```python
from build123d import *

# Parameters (mm, degrees)
BOSS_EXTRU_1_DEPTH           = 23
BOSS_EXTRU_2_DEPTH           = 55.74
ENL_V_MAT_EXTRU_2_DEPTH      = 166.850257131
ENL_V_MAT_EXTRU_2_DEPTH_BACK = 166.850257131
ENL_V_MAT_EXTRU_3_DEPTH      = 172.327320122
ENL_V_MAT_EXTRU_3_DEPTH_BACK = 172.327320122


with BuildPart() as part:
    # Esquisse1 → Boss.-Extru.1 (new body)
    with BuildSketch(Plane.XY):
        with BuildLine():
            Line((39.457988868, 163.966514235), (39.457988868, 111.179894524))
            ThreePointArc((39.457988868, 111.179894524), (40.679417093, 109.678629524), (41.957988868, 108.225722877))
            Line((41.957988868, 108.225722877), (41.957988868, 163.966514235))
            Line((41.957988868, 163.966514235), (39.457988868, 163.966514235))
        make_face()
    extrude(amount=BOSS_EXTRU_1_DEPTH)

    # Esquisse2 → Boss.-Extru.2 (add)
    with BuildSketch(Plane(origin=(0, 163.966514235, 0), x_dir=(1, 0, 0), z_dir=(0, 1, 0))):
        Polygon((41.957988868, 0), (41.957988868, 1.8), (37.657988868, 1.8), (39.457988868, 0), align=None)
        Polygon((41.957988868, -24.8), (41.957988868, -23), (39.457988868, -23), (37.657988868, -24.8), align=None)
    extrude(amount=-BOSS_EXTRU_2_DEPTH)

    # Esquisse4 → Enlèv. mat.-Extru.2 (cut, two sides: drawn at the far end of the back side and taken through both)
    with BuildSketch(Plane.ZY.offset(-39.457988868).offset(-ENL_V_MAT_EXTRU_2_DEPTH_BACK)):
        with BuildLine():
            Line((6.196124825, 159.966514235), (16.73866324, 159.966514235))
            ThreePointArc((16.73866324, 159.966514235), (19.567090365, 158.79494136), (20.73866324, 155.966514235))
            Line((20.73866324, 155.966514235), (20.73866324, 143.19142939))
            ThreePointArc((20.73866324, 143.19142939), (19.567090365, 140.363002265), (16.73866324, 139.19142939))
            Line((16.73866324, 139.19142939), (6.196124825, 139.19142939))
            ThreePointArc((6.196124825, 139.19142939), (3.367697701, 140.363002265), (2.196124825, 143.19142939))
            Line((2.196124825, 143.19142939), (2.196124825, 155.966514235))
            ThreePointArc((2.196124825, 155.966514235), (3.367697701, 158.79494136), (6.196124825, 159.966514235))
        make_face()
        with BuildLine():
            Line((16.73866324, 135.19142939), (6.196124825, 135.19142939))
            ThreePointArc((6.196124825, 135.19142939), (3.367697701, 134.019856515), (2.196124825, 131.19142939))
            Line((2.196124825, 131.19142939), (2.196124825, 119.179894524))
            ThreePointArc((2.196124825, 119.179894524), (3.367697701, 116.351467399), (6.196124825, 115.179894524))
            Line((6.196124825, 115.179894524), (16.73866324, 115.179894524))
            ThreePointArc((16.73866324, 115.179894524), (19.567090365, 116.351467399), (20.73866324, 119.179894524))
            Line((20.73866324, 119.179894524), (20.73866324, 131.19142939))
            ThreePointArc((20.73866324, 131.19142939), (19.567090365, 134.019856515), (16.73866324, 135.19142939))
        make_face()
    extrude(amount=ENL_V_MAT_EXTRU_2_DEPTH + ENL_V_MAT_EXTRU_2_DEPTH_BACK, mode=Mode.SUBTRACT)

    # Esquisse5 → Enlèv. mat.-Extru.3 (cut, two sides: drawn at the far end of the back side and taken through both)
    with BuildSketch(Plane.XY.offset(24.8).offset(-ENL_V_MAT_EXTRU_3_DEPTH_BACK)):
        with BuildLine():
            Line((35.834434648, 116.483137771), (36.387771846, 105.790873255))
            Line((36.387771846, 105.790873255), (45.050231908, 105.102432834))
            ThreePointArc((45.050231908, 105.102432834), (40.024403512, 110.454356706), (35.834434648, 116.483137771))
        make_face()
    extrude(amount=ENL_V_MAT_EXTRU_3_DEPTH + ENL_V_MAT_EXTRU_3_DEPTH_BACK, mode=Mode.SUBTRACT)


solid = part.part
```
Input: part model. Units: mm. Frame: model coordinates. A direction names the side the tool comes from. Coordinates: 2 decimals unless noted, no trailing zeros. Write each loop counter-clockwise with the first axis right and the second up, starting at its lowest first coordinate (ties: lowest second). Pieces come first, ordered by that corner, then holes. Notation, with made-up numbers: M 56.25,58 L 97.25,58 A27 cw 97.25,89 Z; hole C -22,58 d1. An arc over 180 degrees is marked long. Use one line per item in the form item = value.
Q1. Draft query along Z for faces 4 (the face through (41, 135.191, 12)), 5 (the face through (40.73, 116.38, 3.34)), 6 (the face through (40, 136, 24.8)), 7 (the face through (40, 136, -1.8)). Return one class per face: released by +Z, released by -Z, zero draft, split by the parting line, or undercut.
Answer below:
face_4 = undercut
face_5 = undercut
face_6 = released by +Z
face_7 = released by -Z
Q2. Set-up query: faces 1 (the face through (38.55, 137.94, -0.91)), 2 (the face through (41, 115.18, 11)), 3 (the face through (40.217, 110.218, -0.913)). Return all of +Z, -Z, +X, -X, +Y, -Y with unobstructed straight access to the full face (end or side cutting, diameter ignored); none if empty.
Answer below:
face_1 = -X, +Y, -Y
face_2 = +X, -X
face_3 = +Z, -Z, -X, -Y
Q3. Material intervals for probe 1 along Z at (x, y) = (40.85, 147); probe 2 along Y at (x, z) = (41.55, 8.25); probe 3 along X at (y, z) = (118.5, 21.5), sorted ascending. Write a range as from..to.
Answer below:
probe_1 = -1.8..2.2, 20.74..24.8
probe_2 = 108.68..115.18, 135.19..139.19, 159.97..163.97
probe_3 = 39.46..41.96
Q4. Section B-B (y = 124). Return loops of the section in (x, z).
Answer below:
outline = M 37.66,-1.8 L 41.96,-1.8 L 41.96,2.2 L 39.46,2.2 L 39.46,0 Z; M 37.66,24.8 L 39.46,23 L 39.46,20.74 L 41.96,20.74 L 41.96,24.8 Z
Q5. First-contact query: pin 1 (1.2 mm diameter, centred on x = 40.5, z = 14, fed in from -Y); pin 2 (12 mm diameter, centred on y = 122.5, z = 7.5, fed in from -X). Flat tips, straight axial feed; report the tip coordinate or a pass-through.
Answer below:
pin_1 = 109.19
pin_2 = 39.46
Q6. Section D-D (y = 114.5). Return loops of the section in (x, z).
Answer below:
outline = M 37.66,-1.8 L 41.96,-1.8 L 41.96,24.8 L 37.66,24.8 L 39.46,23 L 39.46,0 Z
Q7. Section C-C (x = 38.45). Return loops of the section in (y, z), plus the area to 3 significant figures.
Answer below:
outline = M 112.5,-1.8 L 163.97,-1.8 L 163.97,-1.01 L 112.5,-1.01 Z; M 112.5,24.01 L 163.97,24.01 L 163.97,24.8 L 112.5,24.8 Z
area = 81.5 mm²
Q8. Section A-A (z = 19.25). Return loops of the section in (x, y).
Answer below:
outline = M 39.46,111.18 A50.04 ccw 41.96,108.23 L 41.96,116.07 L 39.46,116.07 Z; M 39.46,134.3 L 41.96,134.3 L 41.96,140.08 L 39.46,140.08 Z; M 39.46,159.08 L 41.96,159.08 L 41.96,163.97 L 39.46,163.97 Z
